CAD build for the part. Positions are in the model's coordinates, mm. A direction names the side the tool comes from. Give positions to 0.01 mm unless a question says otherwise; leave off trailing zeros. Write each loop counter-clockwise with the first axis right and the second up, starting at its lowest first coordinate (ties: lowest second). Pieces come first, ordered by that corner, then holes. Notation, with made-up numbers: (82.5, -2.75) -> (114.5, -2.75) arc R7 ccw to (114.5, 1.25) -> close; hole circle Ø5 at (12, 64). An arc over 180 degrees is marked (long way). Answer as a JSON object with one key per item and string values.
```python
from build123d import *

# Parameters (mm, degrees)
STORE_KASET_L_RAF_1_SAG_1_START = -20
STORE_KASET_L_RAF_1_SAG_1_DEPTH = 735.5


with BuildPart() as part:
    # Sketch1 → STORE_kaset_L_raf_1_sag_1 (new body)
    with BuildSketch(Plane.XY.offset(STORE_KASET_L_RAF_1_SAG_1_START)):
        Polygon((205.5, 404.5), (207.5, 404.5), (207.5, 424.5), (199.5, 424.5), (199.5, 422.5), (205.5, 422.5), align=None)
    extrude(amount=-STORE_KASET_L_RAF_1_SAG_1_DEPTH)


solid = part.part
```
1) Slice it at B-B (y = 411.5). List the corners of the cut face in (x, z), then the cut area to 3 significant figures.
Model answer:
{"outline": "(205.5, -755.5) -> (207.5, -755.5) -> (207.5, -20) -> (205.5, -20) -> close", "area": "1,470 mm2"}
2) 3-axis set-ups, long thin cutter, end or side, ignore diameter. For faces 1 (the flat face through (205.5, 414, -383)), 2 (the flat face through (207.5, 414, -383)): which of +Z, -Z, +X, -X, +Y, -Y reach the whole face in a straight line?
Model answer:
{"face 1": "+Z, -Z, -X, -Y", "face 2": "+Z, -Z, +X, +Y, -Y"}
3) Pin check, flat tips, straight feed: pin 1 (3 mm diameter, centred on x = 202, z = -451, fed in from -Y); pin 2 (5 mm diameter, centred on y = 416.5, z = -571, fed in from -X). Stop position of each tip, or through.
Model answer:
{"pin 1": "stops at y = 422.5", "pin 2": "stops at x = 205.5"}
4) Slice it at C-C (x = 203.25). List the corners of the cut face in (y, z), then the cut area to 3 significant figures.
Model answer:
{"outline": "(422.5, -755.5) -> (424.5, -755.5) -> (424.5, -20) -> (422.5, -20) -> close", "area": "1,470 mm2"}
5) Wall check: probe 1 along Y at (x, z) = (202.5, -656); probe 2 along X at (y, z) = (411.25, -568.5). Give the ranges that are in metal, low to high.
Model answer:
{"probe 1": "y = 422.5 to 424.5", "probe 2": "x = 205.5 to 207.5"}
6) Slice it at A-A (z = -497). List the corners of the cut face in (x, y).
Model answer:
{"outline": "(199.5, 422.5) -> (205.5, 422.5) -> (205.5, 404.5) -> (207.5, 404.5) -> (207.5, 424.5) -> (199.5, 424.5) -> close"}
